Input: part model. Units: mm. Frame: model coordinates. Round coordinates to 2 decimals unless told otherwise and drop trailing zeros. Answer as a JSON object with one key per item and string values.
```python
from build123d import *

# Parameters (mm, degrees)
ESQUISSE1_R             = 20
BOSS_EXTRU_1_DEPTH      = 7.5
CONG_1_R                = 1.7
CONG_3_R                = 1.7
ESQUISSE5_R             = 5
ENL_V_MAT_EXTRU_1_DEPTH = 33.015621312


with BuildPart() as part:
    # Esquisse1 → Boss.-Extru.1 (new, symmetric)
    with BuildSketch(Plane.XY):
        Circle(ESQUISSE1_R)
    extrude(amount=BOSS_EXTRU_1_DEPTH, both=True)

    # Esquisse4 → Enlèvement de matière-Révolution1 (revolve, cut)
    with BuildSketch(Plane(origin=(0, 0, 0), x_dir=(0, 0, -1), z_dir=(1, 0, 0)), mode=Mode.PRIVATE) as enl_vement_de_mati_re_r_volution1_sk:
        Polygon((-5, 20), (-1.324936438, 10), (1.324936438, 10), (5, 20), align=None)
    revolve(enl_vement_de_mati_re_r_volution1_sk.sketch.rotate(Axis((0, 0, 15.788572615), (0, 0, -1)), 90), axis=Axis((0, 0, 15.788572615), (0, 0, -1)), mode=Mode.SUBTRACT)

    # Congé1
    cong_1_edges = [part.edges().sort_by_distance(p)[0] for p in [
        (-10, 0, -1.324936438),
    ]]
    fillet(cong_1_edges, radius=CONG_1_R)

    # Congé3
    cong_3_edges = [part.edges().sort_by_distance(p)[0] for p in [
        (-10, 0, 1.324936438),
    ]]
    fillet(cong_3_edges, radius=CONG_3_R)

    # Esquisse5 → Enlèv. mat.-Extru.1 (cut, through all)
    with BuildSketch(Plane.XY.offset(7.5)):
        Circle(ESQUISSE5_R)
    extrude(amount=-ENL_V_MAT_EXTRU_1_DEPTH, mode=Mode.SUBTRACT)


solid = part.part
```
1) Contact query for flat-ended pins moving along their axis: P1, Ø9, axis at x = 0, y = 0, coming from the -Z side; P2, Ø5, axis at y = -8, z = 5, coming from the -X side. Output: stop coordinate, or through.
Output:
{"P1": "passes through", "P2": "stops at x = -19.23"}
2) Ray query, probe 1 along Z at (x, y) = (-15, 5); probe 2 along Y at (x, z) = (-2.5, 5.25); probe 3 along Z at (x, y) = (5.5, 16). Return the intervals inside material, ascending.
Output:
{"probe 1": "z = -7.5 to -3.46, 3.46 to 7.5", "probe 2": "y = -19.84 to -4.33, 4.33 to 19.84", "probe 3": "z = -7.5 to -3.87, 3.87 to 7.5"}
3) Draft query along Z for faces 1 (the face through (4, -4, 7.5)), 2 (the face through (11.012, -3.468, 1.893)), 3 (the face through (-2.53, 11.392, -1.938)), 4 (the face through (-1.08, -4.88, 0.11)). Return one class per face: +Z half, -Z half, draft (parallel to the pull), parting line (faces both ways), or undercut.
Output:
{"face 1": "+Z half", "face 2": "undercut", "face 3": "undercut", "face 4": "draft"}
